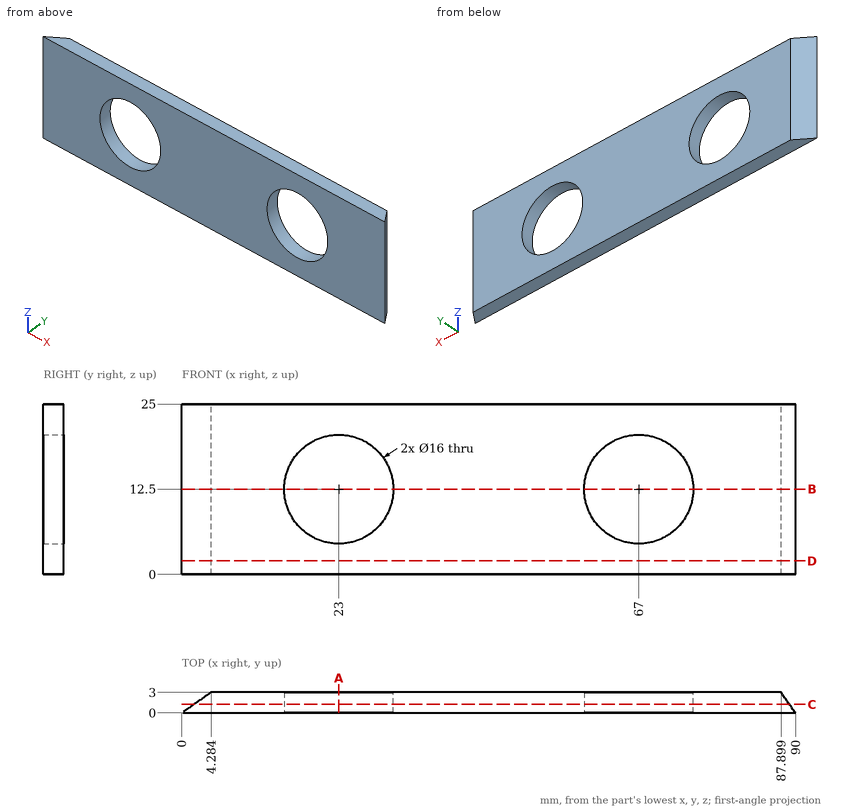
Study the drawing (mm; zero at the part's minimum x, y, z) and answer. Coordinates: 2 decimals unless noted, no trailing zeros. Loops run counter-clockwise (first coordinate to the right, second up) from the corner with the lowest first, then second, coordinate; pieces in that order, holes last. Notation, with made-up numbers: (42.25, 68.25) -> (94.25, 68.25) arc R11 cw to (94.25, 74.25) -> close; hole circle Ø11 at (76, 76). An arc over 180 degrees is marked (long way). Answer as CSV lines item,"result".
1) The part is cut by section C-C (y = 1.25). Give the vertices of the cut face in (x, z) (1 decimal).
A:
outline,"(1.8, 0) -> (89.1, 0) -> (89.1, 25) -> (1.8, 25) -> close; hole circle Ø16 at (23, 12.5); hole circle Ø16 at (67, 12.5)"
2) The part is cut by section A-A (x = 23). Give the vertices of the cut face in (y, z), and give its area (3 significant figures).
A:
outline,"(0, 0) -> (3, 0) -> (3, 4.5) -> (0, 4.5) -> close; (0, 20.5) -> (3, 20.5) -> (3, 25) -> (0, 25) -> close"
area,"27.0 mm²"
3) The part is cut by section D-D (z = 2). Give the vertices of the cut face in (x, y) (1 decimal).
A:
outline,"(0, 0) -> (90, 0) -> (87.9, 3) -> (4.3, 3) -> close"
4) A flat-ended cylindrical pin translates along its axis: pin 1 (14.5 mm diameter, centred on x = 67, z = 12.5, fed in from +Y). Find the tip coordinate at first contact, or state that the pin passes through.
A:
pin 1,"passes through"
5) The part is cut by section B-B (z = 12.5). Give the vertices of the cut face in (x, y) (1 decimal).
A:
outline,"(0, 0) -> (15, 0) -> (15, 3) -> (4.3, 3) -> close; (31, 0) -> (59, 0) -> (59, 3) -> (31, 3) -> close; (75, 0) -> (90, 0) -> (87.9, 3) -> (75, 3) -> close"
6) Straight lines are drawn through the part: probe 1 along Z at (x, y) = (67, 1.1); probe 2 along X at (y, z) = (2.4, 8) (1 decimal); probe 3 along Z at (x, y) = (18.5, 1.35) (1 decimal). For each, find the intervals that lie inside material, in ascending order.
A:
probe 1,"z = 0 to 4.5, 20.5 to 25"
probe 2,"x = 3.4 to 16.4, 29.6 to 60.4, 73.6 to 88.3"
probe 3,"z = 0 to 5.9, 19.1 to 25"
